Model file for the job. Use its own axes, mm. Face numbers are marked on the shaded views. A direction names the side the tool comes from. Give positions to 0.01 mm unless a question says otherwise; leave off trailing zeros. Loops run counter-clockwise (first coordinate to the right, second up) from the corner with the lowest first, then second, coordinate; pieces in that order, holes last. Notation, with made-up numbers: M -11.5,6.25 L 3.5,6.25 A14 cw 3.5,32.25 Z; hole C -11.5,19.25 d3. An arc over 180 degrees is marked long. Answer in a Markdown table with one row per item.
```python
from build123d import *

# Parameters (mm, degrees)
F0_R     = 12.7
F2_DEPTH = 57.15
F1_W     = 127
F1_H     = 50.8
F1_R     = 12.7
F3_DEPTH = 12.7
F4_R     = 5.08
F5_DEPTH = 25.4


with BuildPart() as f2:
    # F0 (on Front) → F2 (new body)
    with BuildSketch(Plane.XZ):
        with BuildLine():
            Line((-31.75, 0), (0, 0))
            Line((0, 0), (31.75, 0))
            Line((31.75, 0), (31.75, 12.7))
            Line((31.75, 12.7), (12.7, 12.7))
            Line((12.7, 12.7), (12.7, 21.59))
            Line((12.7, 21.59), (63.5, 21.59))
            Line((63.5, 21.59), (63.5, 34.29))
            Line((63.5, 34.29), (47.625, 34.29))
            Line((47.625, 34.29), (21.093426, 73.840173))
            ThreePointArc((21.093426, 73.840173), (0, 85.09), (-21.093426, 73.840173))
            Line((-21.093426, 73.840173), (-47.625, 34.29))
            Line((-47.625, 34.29), (-63.5, 34.29))
            Line((-63.5, 34.29), (-63.5, 21.59))
            Line((-63.5, 21.59), (-12.7, 21.59))
            Line((-12.7, 21.59), (-12.7, 12.7))
            Line((-12.7, 12.7), (-31.75, 12.7))
            Line((-31.75, 12.7), (-31.75, 0))
        make_face()
        with Locations((0, 59.69)):
            Circle(F0_R, mode=Mode.SUBTRACT)
    extrude(amount=F2_DEPTH)

    # F1 (on Front) → F3 (join)
    with BuildSketch(Plane.XZ):
        with Locations((0, 59.69)):
            Rectangle(F1_W, F1_H)
        with Locations((0, 59.69)):
            Circle(F1_R, mode=Mode.SUBTRACT)
    extrude(amount=F3_DEPTH)

    # F4 (on face) → F5 (cut)
    with BuildSketch(Plane.XY.offset(85.09)):
        with Locations((0, -34.925)):
            Circle(F4_R)
    extrude(amount=-F5_DEPTH, mode=Mode.SUBTRACT)


solid = f2.part
```
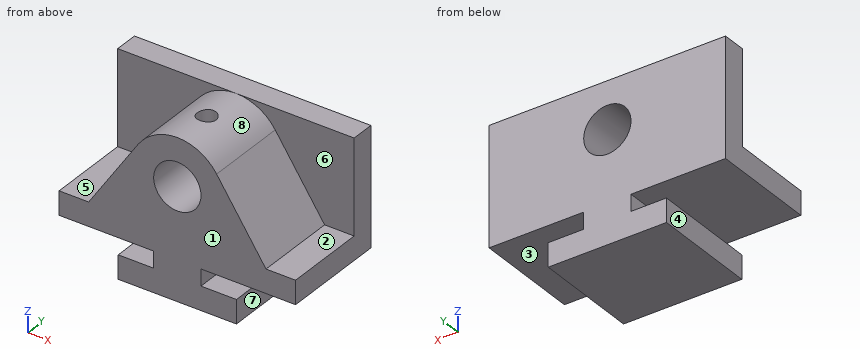
Q1. Mould opens along Z. For the marked faces 1, 2 and 3 say: released by +Z, released by -Z, zero draft, split by the parting line, or undercut.
Reported:
| item | result |
|---|---|
| face 1 | zero draft |
| face 2 | released by +Z |
| face 3 | undercut |
Q2. Saw through at A-A (y = -51). Give the cut face in (x, z) (3 decimals).
Reported:
| item | result |
|---|---|
| outline | M -63.5,21.59 L -12.7,21.59 L -12.7,12.7 L -31.75,12.7 L -31.75,0 L 31.75,0 L 31.75,12.7 L 12.7,12.7 L 12.7,21.59 L 63.5,21.59 L 63.5,34.29 L 47.625,34.29 L 21.093,73.84 A25.4 ccw -21.093,73.84 L -47.625,34.29 L -63.5,34.29 Z; hole C 0,59.69 d25.4 |
Q3. Saw through at B-B (z = 59.69). Give the cut face in (x, y).
Reported:
| item | result |
|---|---|
| outline | M -63.5,-12.7 L -30.59,-12.7 L -30.59,-57.15 L -12.7,-57.15 L -12.7,0 L -63.5,0 Z; M 12.7,-57.15 L 30.59,-57.15 L 30.59,-12.7 L 63.5,-12.7 L 63.5,0 L 12.7,0 Z |
Q4. Probe probe 1 along Z at (x, y) = (0, -26); probe 2 along Y at (x, z) = (0, 80) (3 decimals); probe 3 along Y at (x, z) = (53, 60.5). List the from-to ranges inside material, lowest first.
Reported:
| item | result |
|---|---|
| probe 1 | 0 to 46.99, 72.39 to 85.09 |
| probe 2 | -57.15 to -40.005, -29.845 to 0 |
| probe 3 | -12.7 to 0 |
Q5. 3-axis set-ups, long thin cutter, end or side, ignore diameter. For the marked faces 4, 5, 6, 7 and 8: which of +Z, -Z, +X, -X, +Y, -Y reach the whole face in a straight line?
Reported:
| item | result |
|---|---|
| face 4 | -Z, -X, +Y, -Y |
| face 5 | +Z, -X, -Y |
| face 6 | +Z, +X, -Y |
| face 7 | -Z, +X, +Y, -Y |
| face 8 | +Z, -Y |
Q6. Saw through at C-C (x = 52). Give the cut face in (y, z), and give its area (3 significant figures).
Reported:
| item | result |
|---|---|
| outline | M -57.15,21.59 L 0,21.59 L 0,85.09 L -12.7,85.09 L -12.7,34.29 L -57.15,34.29 Z |
| area | 1,370 mm² |
Q7. Saw through at D-D (y = -5). Give the cut face in (x, z).
Reported:
| item | result |
|---|---|
| outline | M -63.5,21.59 L -12.7,21.59 L -12.7,12.7 L -31.75,12.7 L -31.75,0 L 31.75,0 L 31.75,12.7 L 12.7,12.7 L 12.7,21.59 L 63.5,21.59 L 63.5,85.09 L -63.5,85.09 Z; hole C 0,59.69 d25.4 |
Q8. Drop flat-ended pins along their axis: pin 1 (1.5 mm diameter, centred on x = -31.5, y = -28, fed in from +Z); pin 2 (1 mm diameter, centred on y = -10, z = 14.5, fed in from +X); pin 3 (15 mm diameter, centred on x = 21.5, y = -22.5, fed in from +Z). Give the stop position or say it passes through.
Reported:
| item | result |
|---|---|
| pin 1 | z = 59.45 |
| pin 2 | x = 12.7 |
| pin 3 | z = 80.88 |
